```python
from build123d import *

# Parameters (mm, degrees)
F0_R     = 9.525
F1_DEPTH = 3.81


with BuildPart() as f1:
    # F0 (on Front) → F1 (new body)
    with BuildSketch(Plane.XZ):
        Polygon((57.15, -22.225), (60.96, -22.225), (60.96, 22.225), (57.15, 22.225), (57.15, 13.335), (41.91, 13.335), (41.91, 22.225), (-41.91, 22.225), (-41.91, 13.335), (-57.15, 13.335), (-57.15, 22.225), (-60.96, 22.225), (-60.96, -22.225), (-57.15, -22.225), (-57.15, -13.335), (-41.91, -13.335), (-41.91, -22.225), (41.91, -22.225), (41.91, -13.335), (57.15, -13.335), align=None)
        Circle(F0_R, mode=Mode.SUBTRACT)
    extrude(amount=F1_DEPTH)


solid = f1.part
```
CAD build for the part. Positions are in the model's coordinates, mm. A direction names the side the tool comes from. Coordinates: 2 decimals unless noted, no trailing zeros. Write each loop counter-clockwise with the first axis right and the second up, starting at its lowest first coordinate (ties: lowest second). Pieces come first, ordered by that corner, then holes. Notation, with made-up numbers: (49, 77) -> (90, 77) arc R15 cw to (90, 106) -> close; hole circle Ø10 at (52, 56). An arc over 180 degrees is marked (long way). Return JSON: item names as keys, results as strings. Group by question number.
Q1. Pull direction X, two halves, no side cores. Call faces 1 (the face through (-60.96, -2, 0)), 2 (the face through (59, -2, 22.225)), 3 (the face through (50, -2, 13.335)): released by +X, released by -X, zero draft, split by the parting line, or undercut.
Q2. Flat gauge pin, fed straight in: pin 1 (1.1 mm diameter, centred on x = -50, y = -1.5, fed in from -Z) (3 decimals). Where does the tip first touch, or does it go through?
Q3. Which spindle directions (+Z, -Z, +X, -X, +Y, -Y) get a long thin tool onto all of the face, cutting with end or side? Do faces 4 (the face through (-41.91, -2, -18)), 5 (the face through (-59, -2, -22.225)), 6 (the face through (-57.15, -2, 18)). Say none if no direction does.
Q4. Cut at A-A, the plane x = 0. Give the cut face in (y, z) (3 decimals), then the cut area to 3 significant figures.
Q5. Drill centre lines: line 1 (X direction, y = -2, z = -18); line 2 (Z direction, x = 0, y = -2.05) (3 decimals); line 3 (Z direction, x = -7, y = -3.6) (3 decimals). Where is each one in solid material? Low to high.
Q6. Cut at D-D, the plane z = 0. Give the cut face in (x, y) (3 decimals), then the cut area to 3 significant figures.
Q7. Cut at C-C, the plane y = -1.45. Give the cut face in (x, z) (3 decimals), then the cut area to 3 significant figures.
Q8. Cut at B-B, the plane z = 15. Give the cut face in (x, y).
Returned:
{
 "1": {"face 1": "released by -X", "face 2": "zero draft", "face 3": "undercut"},
 "2": {"pin 1": "stops at z = -13.335"},
 "3": {"face 4": "-Z, +Y, -Y", "face 5": "-Z, +X, -X, +Y, -Y", "face 6": "+Z, +Y, -Y"},
 "4": {"outline": "(-3.81, -22.225) -> (0, -22.225) -> (0, -9.525) -> (-3.81, -9.525) -> close; (-3.81, 9.525) -> (0, 9.525) -> (0, 22.225) -> (-3.81, 22.225) -> close", "area": "96.8 mm2"},
 "5": {"line 1": "x = -60.96 to -57.15, -41.91 to 41.91, 57.15 to 60.96", "line 2": "z = -22.225 to -9.525, 9.525 to 22.225", "line 3": "z = -22.225 to -6.46, 6.46 to 22.225"},
 "6": {"outline": "(-60.96, -3.81) -> (-9.525, -3.81) -> (-9.525, 0) -> (-60.96, 0) -> close; (9.525, -3.81) -> (60.96, -3.81) -> (60.96, 0) -> (9.525, 0) -> close", "area": "392 mm2"},
 "7": {"outline": "(-60.96, -22.225) -> (-57.15, -22.225) -> (-57.15, -13.335) -> (-41.91, -13.335) -> (-41.91, -22.225) -> (41.91, -22.225) -> (41.91, -13.335) -> (57.15, -13.335) -> (57.15, -22.225) -> (60.96, -22.225) -> (60.96, 22.225) -> (57.15, 22.225) -> (57.15, 13.335) -> (41.91, 13.335) -> (41.91, 22.225) -> (-41.91, 22.225) -> (-41.91, 13.335) -> (-57.15, 13.335) -> (-57.15, 22.225) -> (-60.96, 22.225) -> close; hole circle Ø19.05 at (0, 0)", "area": "4,590 mm2"},
 "8": {"outline": "(-60.96, -3.81) -> (-57.15, -3.81) -> (-57.15, 0) -> (-60.96, 0) -> close; (-41.91, -3.81) -> (41.91, -3.81) -> (41.91, 0) -> (-41.91, 0) -> close; (57.15, -3.81) -> (60.96, -3.81) -> (60.96, 0) -> (57.15, 0) -> close"}
}
